For this review, take the finished solid that the model builds, in its own axes (mm). Give positions to 0.01 mm unless a question says otherwise; leave off trailing zeros. Write each loop counter-clockwise with the first axis right and the second up, starting at its lowest first coordinate (ties: lowest second). Pieces come first, ordered by that corner, then holes.
from build123d import *

# Parameters (mm, degrees)
F0_R     = 11.65
F0_R_2   = 3.5
F1_DEPTH = 2.5
F2_DEPTH = 4
F3_DEPTH = 4
F4_DEPTH = 4
F5_DEPTH = 4
F6_DEPTH = 4


with BuildPart() as f1:
    # F0 (on Front) → F1 (new body, symmetric)
    with BuildSketch(Plane.XZ):
        Polygon((0, 33.2328369043), (-65, 33.2328369043), (-65, -33.2328369043), (65, -33.2328369043), (65, 33.2328369043), align=None)
        with Locations((-35, 8.2328369043)):
            Circle(F0_R, mode=Mode.SUBTRACT)
        with Locations((-11.6665, 8.2328369043)):
            Circle(F0_R, mode=Mode.SUBTRACT)
        with Locations((11.667, 8.2328369043)):
            Circle(F0_R, mode=Mode.SUBTRACT)
        with Locations((35, 8.2328369043)):
            Circle(F0_R, mode=Mode.SUBTRACT)
        with Locations((-11.6665, 8.2328369043)):
            Circle(F0_R)
        with Locations((-11.6665, 8.2328369043)):
            Circle(F0_R_2, mode=Mode.SUBTRACT)
        with Locations((11.667, 8.2328369043)):
            Circle(F0_R)
        with Locations((11.667, 8.2328369043)):
            Circle(F0_R_2, mode=Mode.SUBTRACT)
        with Locations((35, 8.2328369043)):
            Circle(F0_R)
        with Locations((35, 8.2328369043)):
            Circle(F0_R_2, mode=Mode.SUBTRACT)
        with Locations((-35, 8.2328369043)):
            Circle(F0_R)
        with Locations((-35, 8.2328369043)):
            Circle(F0_R_2, mode=Mode.SUBTRACT)
    extrude(amount=F1_DEPTH, both=True)

    # F0 (on Front) → F2 (join)
    with BuildSketch(Plane.XZ):
        with Locations((35, 8.2328369043)):
            Circle(F0_R)
        with Locations((35, 8.2328369043)):
            Circle(F0_R_2, mode=Mode.SUBTRACT)
    extrude(amount=F2_DEPTH)

    # F0 (on Front) → F3 (join)
    with BuildSketch(Plane.XZ):
        with Locations((-35, 8.2328369043)):
            Circle(F0_R)
        with Locations((-35, 8.2328369043)):
            Circle(F0_R_2, mode=Mode.SUBTRACT)
    extrude(amount=F3_DEPTH)

    # F0 (on Front) → F4 (join)
    with BuildSketch(Plane.XZ):
        with Locations((-11.6665, 8.2328369043)):
            Circle(F0_R)
        with Locations((-11.6665, 8.2328369043)):
            Circle(F0_R_2, mode=Mode.SUBTRACT)
    extrude(amount=F4_DEPTH)

    # F0 (on Front) → F5 (join)
    with BuildSketch(Plane.XZ):
        with Locations((11.667, 8.2328369043)):
            Circle(F0_R)
        with Locations((11.667, 8.2328369043)):
            Circle(F0_R_2, mode=Mode.SUBTRACT)
    extrude(amount=F5_DEPTH)

    # F0 (on Front) → F6 (join)
    with BuildSketch(Plane.XZ):
        with Locations((11.667, 8.2328369043)):
            Circle(F0_R)
        with Locations((11.667, 8.2328369043)):
            Circle(F0_R_2, mode=Mode.SUBTRACT)
    extrude(amount=F6_DEPTH)


solid = f1.part
(1) We need section D-D (x = -17). Write out the cut boundary in (y, z), and give its area (3 significant figures).
(2) We need section A-A (x = 35). Write out the cut boundary in (y, z).
(3) We need section C-C (z = -22). Write out the cut boundary in (x, y), and give its area (3 significant figures).
(4) We need section B-B (y = -1.5). Write out the cut boundary in (x, z), and give its area (3 significant figures).
(5) Clearance check with flat-ended pins moving along their axes: pin 1 Ø6.5 at (x, z) = (-11.67, 8.23) entering from -Y; pin 2 Ø11 at (x, z) = (-35, 8.23) entering from +Y. State where each tip first meets the part, or that it passes through.
(6) For L1, parallel to Z at x = 35, y = -0.75; L2, parallel to Z at x = 35, y = -3.5; L3, parallel to Y at x = 51, z = -18, list the stretches that pass through material, from the lowest coordinate up.
(7) The part is to be moulded in two halves that separate along Z. For faces 1 (the flat face through (1, 0, 33.233)), 2 (the flat face through (-1, 0, -33.233)), 3 (the flat face through (-65, 0, 0)), 4 (the cylindrical face through (8.17, -0.7, 8.39)), say which applies: +Z half, -Z half, draft (parallel to the pull), parting line (faces both ways), or undercut.
The answers:
1. outline: (-4, -2.12) - (-2.5, -2.12) - (-2.5, -33.23) - (2.5, -33.23) - (2.5, 33.23) - (-2.5, 33.23) - (-2.5, 18.59) - (-4, 18.59) - close
1. area: 363 mm2
2. outline: (-4, -3.42) - (-2.5, -3.42) - (-2.5, -33.23) - (2.5, -33.23) - (2.5, 4.73) - (-4, 4.73) - close; (-4, 11.73) - (2.5, 11.73) - (2.5, 33.23) - (-2.5, 33.23) - (-2.5, 19.88) - (-4, 19.88) - close
3. outline: (-65, -2.5) - (65, -2.5) - (65, 2.5) - (-65, 2.5) - close
3. area: 650 mm2
4. outline: (-65, -33.23) - (65, -33.23) - (65, 33.23) - (-65, 33.23) - close; hole circle Ø7 at (-35, 8.23); hole circle Ø7 at (-11.67, 8.23); hole circle Ø7 at (11.67, 8.23); hole circle Ø7 at (35, 8.23)
4. area: 8,490 mm2
5. pin 1: passes through
5. pin 2: stops at y = 2.5
6. L1: z = -33.23 to 4.73, 11.73 to 33.23
6. L2: z = -3.42 to 4.73, 11.73 to 19.88
6. L3: y = -2.5 to 2.5
7. face 1: +Z half
7. face 2: -Z half
7. face 3: draft
7. face 4: undercut
